Study the drawing (mm; zero at the part's minimum x, y, z) and answer. Coordinates: 2 decimals unless noted, no trailing zeros. Write each loop counter-clockwise with the first axis right and the second up, starting at its lowest first coordinate (ties: lowest second). Pieces come first, ordered by that corner, then holes. Notation, with made-up numbers: M 36,19.25 L 95,19.25 A14 cw 95,34.25 Z; hole C 82,89.5 d4. An arc over 180 degrees is marked long. Answer as CSV lines item,"result". Start each with the question number.
(1) A cutting plane is placed at B-B on z = 177. Give the vertices of the cut face in (x, y).
(2) A cutting plane is placed at D-D on z = 74. Give the vertices of the cut face in (x, y), then the cut area to 3 significant figures.
(3) Flat-ended cylindrical pins translate along their axes: P1, Ø4, axis at y = 3, z = 40, coming from the +X side; P2, Ø2, axis at x = 6.5, z = 31, coming from the -Y side. Find the tip coordinate at first contact, or state that the pin passes through.
(4) A cutting plane is placed at A-A on x = 10.65. Give the vertices of the cut face in (y, z).
(5) A cutting plane is placed at C-C on y = 10.65. Give the vertices of the cut face in (x, z), then the cut area to 3 significant figures.
(6) Find the intervals of material crossed by L1, parallel to Y at x = 10.65, z = 110.5; L2, parallel to Y at x = 3.5, z = 37.5; L3, parallel to X at y = 9.75, z = 203, in increasing order. Write a range as [from, to].
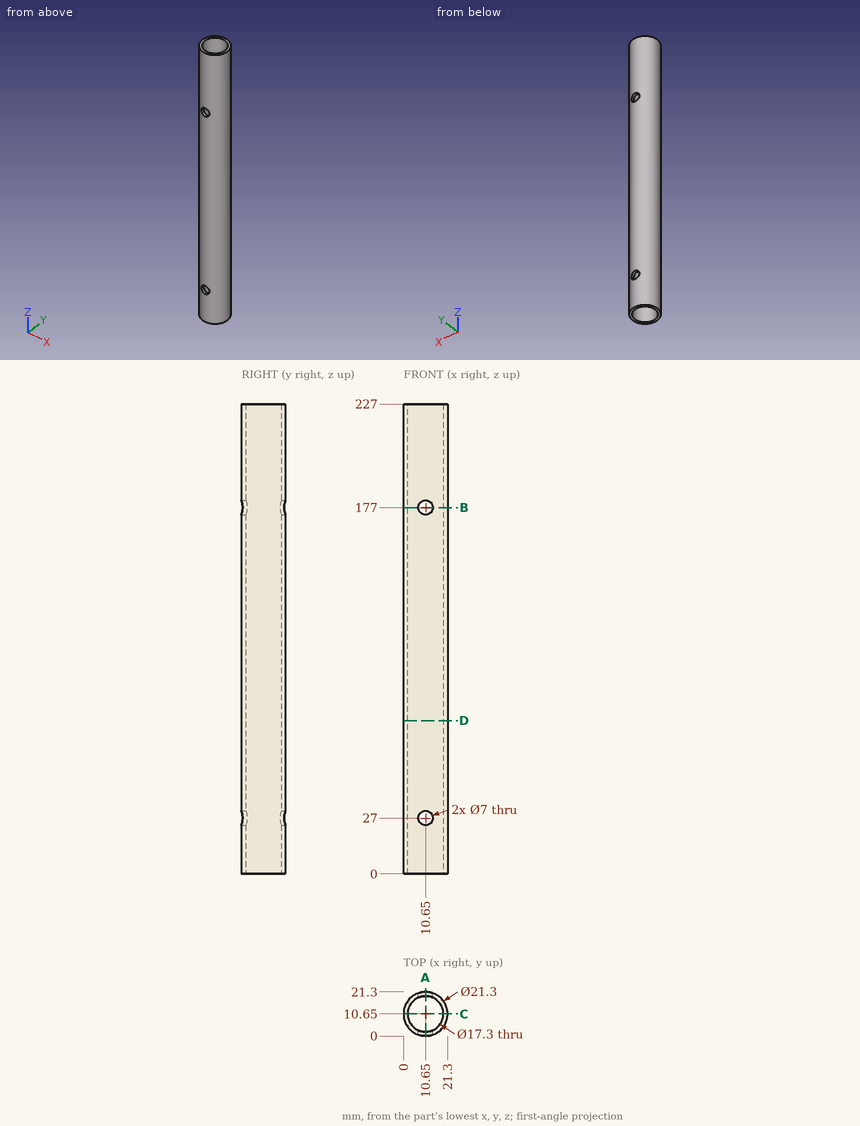
Here are the results:
1,outline,"M 7.15,0.59 L 7.15,2.74 A8.65 cw 7.15,18.56 L 7.15,20.71 A10.65 ccw Z; M 14.15,0.59 A10.65 ccw 14.15,20.71 L 14.15,18.56 A8.65 cw 14.15,2.74 Z"
2,outline,"C 10.65,10.65 d21.3; hole C 10.65,10.65 d17.3"
2,area,"121 mm^2"
3,P1,"stops at x = 19.68"
3,P2,"stops at y = 0.48"
4,outline,"M 0,0 L 2,0 L 2,23.5 L 0,23.5 Z; M 0,30.5 L 2,30.5 L 2,173.5 L 0,173.5 Z; M 0,180.5 L 2,180.5 L 2,227 L 0,227 Z; M 19.3,0 L 21.3,0 L 21.3,23.5 L 19.3,23.5 Z; M 19.3,30.5 L 21.3,30.5 L 21.3,173.5 L 19.3,173.5 Z; M 19.3,180.5 L 21.3,180.5 L 21.3,227 L 19.3,227 Z"
5,outline,"M 0,0 L 2,0 L 2,227 L 0,227 Z; M 19.3,0 L 21.3,0 L 21.3,227 L 19.3,227 Z"
5,area,"908 mm^2"
6,L1,"y = [0, 2], [19.3, 21.3]"
6,L2,"y = [2.76, 5.78], [15.52, 18.54]"
6,L3,"x = [0.04, 2.05], [19.25, 21.26]"
